The model under review builds one solid part; all positions refer to its coordinate system, in mm. Face numbers are marked on the shaded views. A direction names the side the tool comes from. Coordinates: 2 decimals unless noted, no trailing zeros. Write each loop counter-clockwise with the first axis right and the second up, starting at its lowest first coordinate (ties: lowest second). Pieces come first, ordered by that corner, then holes. Notation, with made-up numbers: (29, 47) - (81, 47) arc R24 cw to (81, 64) - close; hole circle Ø2 at (61.25, -16.5). An arc over 180 degrees is marked (long way). Put each result on its own line as item: value.
from build123d import *

# Parameters (mm, degrees)
THICKEN_1_T2        = 2
SKETCH_2_R          = 29.732137495
EXTRUDE_1_DEPTH     = 2
SKETCH_2_3_W        = 8.7
SKETCH_2_3_H        = 8.7
CUT_EXTRUDE_1_DEPTH = 59.86436084


with BuildPart() as body_1:
    # Sheet Revolve 1: a surface, the sketch's curves turned about an axis
    with BuildLine(Plane.XY, mode=Mode.PRIVATE) as sheet_revolve_1_1_path:
        Line((34.75, 8.5), (29.732137495, 8.5))
        ThreePointArc((29.732137495, 8.5), (27.09901514, 9.488909389), (25.767852495, 11.966666667))
        ThreePointArc((25.767852495, 11.966666667), (25.354764169, 14.256382016), (24.738633754, 16.5))
    sheet_revolve_1_1 = Shell.revolve(sheet_revolve_1_1_path.wire(), 360, Axis((0, 50, 0), (0, -1, 0)))
    add(Solid.thicken(sheet_revolve_1_1, -THICKEN_1_T2))

    # Sketch 2 → Extrude 1 (add)
    with BuildSketch(Plane.XZ.offset(-8.5)):
        with BuildLine():
            Line((-23.614933424, 25.493085717), (-43.727741416, 6.862048778))
            ThreePointArc((-43.727741416, 6.862048778), (-46.725, 0), (-43.727741416, -6.862048778))
            Line((-43.727741416, -6.862048778), (-23.614933424, -25.493085717))
            ThreePointArc((-23.614933424, -25.493085717), (0, -34.75), (23.614933424, -25.493085717))
            Line((23.614933424, -25.493085717), (43.727741416, -6.862048778))
            ThreePointArc((43.727741416, -6.862048778), (46.725, 0), (43.727741416, 6.862048778))
            Line((43.727741416, 6.862048778), (23.614933424, 25.493085717))
            ThreePointArc((23.614933424, 25.493085717), (0, 34.75), (-23.614933424, 25.493085717))
        make_face()
        Circle(SKETCH_2_R, mode=Mode.SUBTRACT)
    extrude(amount=-EXTRUDE_1_DEPTH)

    # Sketch 2_3 → Cut-Extrude 1 (cut, through all)
    with BuildSketch(Plane.XZ.offset(-8.5)):
        with Locations((-37.675, 0)):
            Rectangle(SKETCH_2_3_W, SKETCH_2_3_H)
        with Locations((37.675, 0)):
            Rectangle(SKETCH_2_3_W, SKETCH_2_3_H)
    extrude(amount=-CUT_EXTRUDE_1_DEPTH, mode=Mode.SUBTRACT)


solid = body_1.part
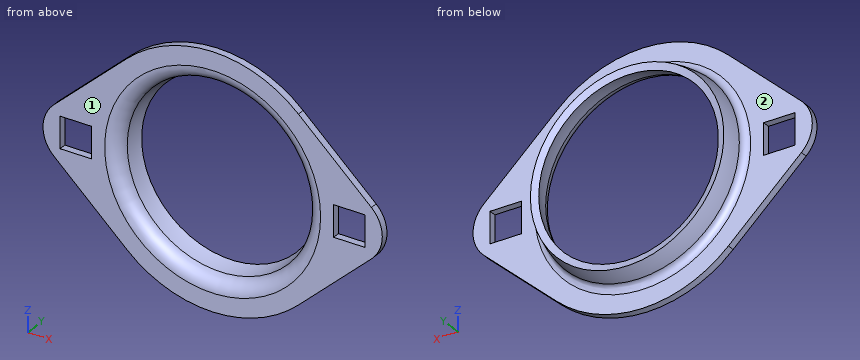
1. Consider section A-A on z = 0. State the section outline as (x, y) points (3 decimals), plus the area to 3 significant figures.
Determined:
outline: (-46.725, 8.5) - (-42.025, 8.5) - (-42.025, 10.5) - (-46.725, 10.5) - close; (-33.325, 8.5) - (-29.732, 8.5) arc R4 ccw to (-25.768, 11.967) arc R26 cw to (-24.739, 16.5) - (-26.642, 17.115) arc R28 ccw to (-27.75, 12.233) arc R2 cw to (-29.732, 10.5) - (-33.325, 10.5) - close; (24.739, 16.5) arc R26 cw to (25.768, 11.967) arc R4 ccw to (29.732, 8.5) - (33.325, 8.5) - (33.325, 10.5) - (29.732, 10.5) arc R2 cw to (27.75, 12.233) arc R28 ccw to (26.642, 17.115) - close; (42.025, 8.5) - (46.725, 8.5) - (46.725, 10.5) - (42.025, 10.5) - close
area: 69.8 mm^2
2. Machinability: for the marked faces 1 and 2, which of the approach directions +Z, -Z, +X, -X, +Y, -Y give a long, thin tool a straight path to every point of the face, cutting with its end or side? Answer none if there is none.
Determined:
face 1: +Z, -Z, +X, -X, -Y
face 2: +Y
3. For pin 1 Ø5 at (x, z) = (-30.5, 3.5) entering from +Y; pin 2 Ø5 at (y, z) = (10, -21) entering from +X; pin 3 Ø2 at (y, z) = (9, 2) entering from +X, all flat-tipped, find the tip position at first contact; note any pin that passes through.
Determined:
pin 1: stops at y = 11.21
pin 2: stops at x = 31.16
pin 3: stops at x = 46.67
4. To check wall thickness, follow probe 1 along X at (y, z) = (9.75, 2) (3 decimals); probe 2 along Y at (x, z) = (-35, -5.5); probe 3 along Z at (x, y) = (14.5, 15.5). State the ranges of each line that lie inside material, in increasing order.
Determined:
probe 1: x = -46.509 to -42.025, -33.325 to -26.753, 26.753 to 33.325, 42.025 to 46.509
probe 2: y = 8.5 to 10.5
probe 3: z = -22.91 to -20.41, 20.41 to 22.91
5. Consider section C-C on y = 15.5. State the section outline as (x, z) points, plus the area to 3 significant figures.
Determined:
outline: circle Ø54.22 at (0, 0); hole circle Ø50.08 at (0, 0)
area: 339 mm^2
6. Consider section B-B on x = 0. State the section outline as (y, z) points.
Determined:
outline: (8.5, -34.75) - (10.5, -34.75) - (10.5, -29.73) arc R2 cw to (12.23, -27.75) arc R28 ccw to (17.12, -26.64) - (16.5, -24.74) arc R26 cw to (11.97, -25.77) arc R4 ccw to (8.5, -29.73) - close; (8.5, 29.73) arc R4 ccw to (11.97, 25.77) arc R26 cw to (16.5, 24.74) - (17.12, 26.64) arc R28 ccw to (12.23, 27.75) arc R2 cw to (10.5, 29.73) - (10.5, 34.75) - (8.5, 34.75) - close
